For this review, take the finished solid that the model builds, in its own axes (mm). A direction names the side the tool comes from. Coordinates: 2 decimals unless noted, no trailing zeros. Write each loop counter-clockwise with the first axis right and the second up, starting at its lowest first coordinate (ties: lowest second). Pieces come first, ordered by that corner, then holes.
Autodesk Fusion 360 part; units mm, degrees
sketch "Sketch1" plane through (0, 0, 0) normal (1, 0, 0) x (0, 1, 0)
  line L0 (-125, 0) -> (375, 0)
  dimension "d1" = 500
sketch "Sketch4" plane through (0, 0, 0) normal (0, 1, 0) x (1, 0, 0)
  line L0 (2.79, 7.645) -> (-7.71, 7.645)
  line L1 (-7.71, 7.645) -> (-7.71, -2.855)
  line L2 (-7.71, -2.855) -> (2.79, -2.855)
  line L3 (2.79, -2.855) -> (2.79, 7.645)
  line L4 (2.79, 7.645) -> (-7.71, -2.855) construction
  line L5 (-7.71, 7.645) -> (2.79, -2.855) construction
  line L6 (1.79, 6.645) -> (-6.71, 6.645)
  line L7 (-6.71, 6.645) -> (-6.71, -1.855)
  line L8 (-6.71, -1.855) -> (1.79, -1.855)
  line L9 (1.79, -1.855) -> (1.79, 6.645)
  line L10 (1.79, 6.645) -> (-6.71, -1.855) construction
  line L11 (-6.71, 6.645) -> (1.79, -1.855) construction
  point P0 (-2.46, 2.395)
  point P1 (-2.46, 2.395)
  dimension "d2" = 10.5
  dimension "d3" = 10.5
  dimension "d4" = 8.5
  dimension "d5" = 8.5
sweep "Sweep1" add profiles "Sketch4" path "Sketch1" along L0 section 1
1) Consider section C-C (x = -4.75). Give the boundary of the cut face in (y, z) (3 decimals), then the cut area to 3 significant figures.
2) The part is to be moulded in two halves that separate along X. For faces 3 (the face through (-7.71, 128, -2)), 4 (the face through (-6.71, 128, -2)), 5 (the face through (-3, 128, -6.645)), 6 (the face through (-3, 128, 2.855)), say which applies: pulls with the +X half, pulls with the -X half, needs draft (parallel to the pull), parting line crosses it, or undercut.
3) Consider section A-A (z = -2). Give the boundary of the cut face in (x, y), then the cut area to 3 significant figures.
4) For L1, parallel to Z at x = -6, y = 87 (3 decimals); L2, parallel to X at y = 170.5, z = -4.5, list the stretches that pass through material, from the lowest coordinate up.
5) Tool access review of faces 1 (the face through (-2, 128, 1.855)), 2 (the face through (-2, 375, -7)): name each direction out of +Z, -Z, +X, -X, +Y, -Y from which nothing blocks a thin tool from reaching the whole face with its end or side.
6) Consider section B-B (y = 158). Give the boundary of the cut face in (x, z) (3 decimals), then the cut area to 3 significant figures.
Results:
1. outline: (-125, -7.645) - (375, -7.645) - (375, -6.645) - (-125, -6.645) - close; (-125, 1.855) - (375, 1.855) - (375, 2.855) - (-125, 2.855) - close
1. area: 1,000 mm2
2. face 3: pulls with the -X half
2. face 4: undercut
2. face 5: undercut
2. face 6: needs draft
3. outline: (-7.71, -125) - (-6.71, -125) - (-6.71, 375) - (-7.71, 375) - close; (1.79, -125) - (2.79, -125) - (2.79, 375) - (1.79, 375) - close
3. area: 1,000 mm2
4. L1: z = -7.645 to -6.645, 1.855 to 2.855
4. L2: x = -7.71 to -6.71, 1.79 to 2.79
5. face 1: +Y, -Y
5. face 2: +Z, -Z, +X, -X, +Y
6. outline: (-7.71, -7.645) - (2.79, -7.645) - (2.79, 2.855) - (-7.71, 2.855) - close; hole (-6.71, -6.645) - (1.79, -6.645) - (1.79, 1.855) - (-6.71, 1.855) - close
6. area: 38.0 mm2
